from build123d import *

# Parameters (mm, degrees)
PAD_DEPTH       = 5
SKETCH001_W     = 29
SKETCH001_H     = 16
POCKET_DEPTH    = 5
SKETCH002_W     = 29
SKETCH002_H     = 2.2
POCKET001_DEPTH = 2.1
POCKET002_DEPTH = 100
POCKET003_DEPTH = 100
SKETCH006_W     = 3
SKETCH006_H     = 5
SKETCH006_W_2   = 6
PAD001_DEPTH    = 5.5
SKETCH008_W     = 2.2
SKETCH008_H     = 5.7
POCKET005_DEPTH = 5
SKETCH009_R     = 0.75
POCKET006_DEPTH = 200
FILLET_R        = 2.49


with BuildPart() as part:
    # Sketch → Pad (new body)
    with BuildSketch(Plane.XY):
        Polygon((-85, 14), (85, 14), (78.535691, -14), (-91.464309, -14), align=None)
    extrude(amount=PAD_DEPTH)

    # Sketch001 (on Face6 of Pad) → Pocket (cut)
    with BuildSketch(Plane.XY.offset(5)):
        with Locations((0, -6)):
            Rectangle(SKETCH001_W, SKETCH001_H)
    extrude(amount=-POCKET_DEPTH, mode=Mode.SUBTRACT)

    # Sketch002 (on Face9 of Pocket) → Pocket001 (cut)
    with BuildSketch(Plane.XZ.offset(-2)):
        with Locations((0, 2.5)):
            Rectangle(SKETCH002_W, SKETCH002_H)
    extrude(amount=-POCKET001_DEPTH, mode=Mode.SUBTRACT)

    # Sketch004 (on Face8 of Pocket001) → Pocket002 (cut)
    with BuildSketch(Plane.YZ.offset(-14.5)):
        Polygon((-14, 5), (2, 5), (-14, 3), align=None)
    extrude(amount=-POCKET002_DEPTH, mode=Mode.SUBTRACT)

    # Sketch005 (on Face11 of Pocket002) → Pocket003 (cut)
    with BuildSketch(Plane(origin=(14.5, 0, 0), x_dir=(0, -1, 0), z_dir=(-1, 0, 0))):
        Polygon((-2, 5), (14, 5), (14, 3), align=None)
    extrude(amount=-POCKET003_DEPTH, mode=Mode.SUBTRACT)

    # Sketch006 (on Face1 of Pocket003) → Pad001 (join)
    with BuildSketch(Plane(origin=(0, 14, 0), x_dir=(-1, 0, 0), z_dir=(0, 1, 0))):
        with Locations((83.5, 2.5)):
            Rectangle(SKETCH006_W, SKETCH006_H)
        with Locations((-83.5, 2.5)):
            Rectangle(SKETCH006_W, SKETCH006_H)
        with Locations((0, 2.5)):
            Rectangle(SKETCH006_W_2, SKETCH006_H)
    extrude(amount=PAD001_DEPTH)

    # Sketch008 (on Face5 of Pocket001) → Pocket005 (cut)
    with BuildSketch(Plane.XY.offset(5)):
        with Locations((-41.1, 7.15)):
            Rectangle(SKETCH008_W, SKETCH008_H)
    extrude(amount=-POCKET005_DEPTH, mode=Mode.SUBTRACT)

    # Sketch009 (on Face35 of Pocket005) → Pocket006 (cut)
    with BuildSketch(Plane.YZ.offset(85)):
        with Locations((17, 2.5)):
            Circle(SKETCH009_R)
    extrude(amount=-POCKET006_DEPTH, mode=Mode.SUBTRACT)

    # Fillet
    fillet_edges = [part.edges().sort_by_distance(p)[0] for p in [
        (83.5, 19.5, 5),
        (83.5, 19.5, 0),
        (0, 19.5, 5),
        (0, 19.5, 0),
        (-83.5, 19.5, 5),
        (-83.5, 19.5, 0),
    ]]
    fillet(fillet_edges, radius=FILLET_R)


solid = part.part
Input: part model. Units: mm. Frame: model coordinates. A direction names the side the tool comes from. Give positions to 0.01 mm unless a question says otherwise; leave off trailing zeros. Write each loop counter-clockwise with the first axis right and the second up, starting at its lowest first coordinate (ties: lowest second). Pieces come first, ordered by that corner, then holes. Notation, with made-up numbers: (84, 83) -> (110, 83) arc R26 cw to (110, 107) -> close; hole circle Ø11 at (-1.5, 9). An arc over 180 degrees is marked (long way). Use one line per item in the form item = value. Start each with the question number.
1) Ray query, probe 1 along X at (y, z) = (18.5, 4.2); probe 2 along Z at (x, y) = (83, 17); probe 3 along X at (y, z) = (2, 1.95). Return the intervals inside material, ascending. Write a range as from..to.
2) Set-up query: faces 1 (the flat face through (-85, 16, 2)), 2 (the flat face through (42, 14, 2)), 3 (the flat face through (-42.2, 7, 3)). Return all of +Z, -Z, +X, -X, +Y, -Y with unobstructed straight access to the full face (end or side cutting, diameter ignored); none if empty.
3) Pin query (flat end, axial travel): pin 1 (1.5 mm diameter, centred on y = 6.5, z = 3, fed in from +X); pin 2 (0.9 mm diameter, centred on y = 17, z = 2.5, fed in from -X); pin 3 (1.5 mm diameter, centred on x = -45.5, z = 1, fed in from +Y); pin 4 (0.7 mm diameter, centred on x = -2, z = 4.5, fed in from -Y). Return the tip coordinate at first contact, or that it passes through.
4) Section query C-C on x = -18. Return the cut outline in (y, z).
5) Section query B-B on y = 6. Return the cut outline in (x, z).
6) Draft query along X for faces 4 (the flat face through (-3, 16, 2)), 5 (the flat face through (48, -6, 4)), 6 (the flat face through (-88.28, -0.2, 2.46)). Return one class per face: pulls with the +X half, pulls with the -X half, needs draft (parallel to the pull), parting line crosses it, or undercut.
Outcome:
q1.probe_1 = -85..-82, -3..3, 82..85
q1.probe_2 = 0..1.75, 3.25..5
q1.probe_3 = -87.77..-14.5, 14.5..82.23
q2.face_1 = +Z, -Z, -X, +Y
q2.face_2 = +Z, -Z, +Y
q2.face_3 = +Z, -Z
q3.pin_1 = 83.44
q3.pin_2 = through
q3.pin_3 = 14
q3.pin_4 = 2
q4.outline = (-14, 0) -> (14, 0) -> (14, 5) -> (2, 5) -> (-14, 3) -> close
q5.outline = (-86.85, 0) -> (-42.2, 0) -> (-42.2, 5) -> (-86.85, 5) -> close; (-40, 0) -> (83.15, 0) -> (83.15, 5) -> (-40, 5) -> close
q6.face_4 = undercut
q6.face_5 = needs draft
q6.face_6 = pulls with the -X half
